from build123d import *

# Parameters (mm, degrees)
BOSS_EXTRUDE2_DEPTH      = 5
BOSS_EXTRUDE2_DEPTH_BACK = 5
CUT_EXTRUDE1_DEPTH       = 33.786759245
CUT_EXTRUDE1_DEPTH_BACK  = 33.786759245
SKETCH2_R                = 2
BOSS_EXTRUDE3_DEPTH      = 5
BOSS_EXTRUDE3_DEPTH_BACK = 5
SKETCH3_W                = 8
SKETCH3_H                = 1.5
CUT_EXTRUDE2_DEPTH       = 32.24718732
CUT_EXTRUDE2_DEPTH_BACK  = 32.24718732
SKETCH4_R                = 2
FILLET1_R                = 3


with BuildPart() as part:
    # Sketch1 → Boss-Extrude2 (new, two sides: drawn at the far end of the back side and taken through both)
    with BuildSketch(Plane.XY.offset(-BOSS_EXTRUDE2_DEPTH_BACK)):
        with BuildLine():
            Line((-16.929532322, 1.5), (-24.929532322, 1.5))
            Line((-24.929532322, 1.5), (-24.929532322, 3.5))
            Line((-24.929532322, 3.5), (-17.840130641, 3.5))
            ThreePointArc((-17.840130641, 3.5), (-10.970967291, 14.01498524), (1.215, 17.05678091))
            ThreePointArc((1.215, 17.05678091), (17.1, 0), (1.215, -17.05678091))
            ThreePointArc((1.215, -17.05678091), (-10.970967291, -14.01498524), (-17.840130641, -3.5))
            Line((-17.840130641, -3.5), (-24.929532322, -3.5))
            Line((-24.929532322, -3.5), (-24.929532322, -1.5))
            Line((-24.929532322, -1.5), (-16.929532322, -1.5))
            ThreePointArc((-16.929532322, -1.5), (-10.970813778, -12.51330782), (1.095, -15.862249998))
            ThreePointArc((1.095, -15.862249998), (15.9, 0), (1.095, 15.862249998))
            ThreePointArc((1.095, 15.862249998), (-10.970813778, 12.51330782), (-16.929532322, 1.5))
        make_face()
    extrude(amount=BOSS_EXTRUDE2_DEPTH + BOSS_EXTRUDE2_DEPTH_BACK)

    # Sketch2 → Cut-Extrude1 (cut, two sides: drawn at the far end of the back side and taken through both)
    with BuildSketch(Plane(origin=(0, 3.5, 0), x_dir=(1, 0, 0), z_dir=(0, 1, 0)).offset(-CUT_EXTRUDE1_DEPTH_BACK)):
        with Locations(Location((-21.429532322, 0, 0), (0, 0, 180))):
            Circle(SKETCH2_R)
    extrude(amount=CUT_EXTRUDE1_DEPTH + CUT_EXTRUDE1_DEPTH_BACK, mode=Mode.SUBTRACT)

    # Sketch3 → Boss-Extrude3 (add, two sides: drawn at the far end of the back side and taken through both)
    with BuildSketch(Plane.XY.offset(-BOSS_EXTRUDE3_DEPTH_BACK)):
        with Locations((21.083544714, 0)):
            Rectangle(SKETCH3_W, SKETCH3_H)
    extrude(amount=BOSS_EXTRUDE3_DEPTH + BOSS_EXTRUDE3_DEPTH_BACK)

    # Sketch4 → Cut-Extrude2 (cut, two sides: drawn at the far end of the back side and taken through both)
    with BuildSketch(Plane(origin=(0, 0.75, 0), x_dir=(1, 0, 0), z_dir=(0, 1, 0)).offset(-CUT_EXTRUDE2_DEPTH_BACK)):
        with Locations(Location((21.083544714, 0, 0), (0, 0, 180))):
            Circle(SKETCH4_R)
    extrude(amount=CUT_EXTRUDE2_DEPTH + CUT_EXTRUDE2_DEPTH_BACK, mode=Mode.SUBTRACT)

    # Fillet1
    fillet1_edges = [part.edges().sort_by_distance(p)[0] for p in [
        (-24.929532322, -2.5, -5),
        (-24.929532322, -2.5, 5),
        (-24.929532322, 2.5, 5),
        (-24.929532322, 2.5, -5),
        (25.083544714, 0, -5),
        (25.083544714, 0, 5),
    ]]
    fillet(fillet1_edges, radius=FILLET1_R)


solid = part.part
Could you check a few things on this model? Use its own coordinates, in mm. A direction names the side the tool comes from. Give positions to 0.01 mm unless a question says otherwise; leave off trailing zeros. Order: outer loops, then holes, each group sorted by start corner. A loop starts at its lowest first (then second) coordinate and runs counter-clockwise, first axis right, second up. Notation, with made-up numbers: (66, 38) -> (113, 38) arc R23 ccw to (113, 70) -> close; hole circle Ø8 at (-37.75, -28). An arc over 180 degrees is marked (long way). Answer in a Markdown table with one row per item. Add a question column.
Item 1: Imagine slicing it at B-B (z = 0). List the corners of the cut face in (x, y) for me (3 decimals).
Item 2: For faces 1 (the cylindrical face through (15.896, -0.334, -0.07)), 2 (the flat face through (-19, -1.5, 0)), 3 (the flat face through (-21.3, -3.5, 2.2)), 4 (the flat face through (-19, 3.5, 0)), which set-ups out of +Z, -Z, +X, -X, +Y, -Y let a thin tool reach every point of the face, with its end or its side?
Item 3: Imagine slicing it at D-D (y = 15). List the corners of the cut face in (x, z) for me, and give its area (3 significant figures).
Item 4: Please list where these lines run through material, in increasing order: probe 1 along X at (y, z) = (-2.2, 0); probe 2 along X at (y, z) = (-2.55, 0); probe 3 along Y at (x, z) = (1, 0.75).
Item 5: Imagine slicing it at C-C (x = 9.5). List the corners of the cut face in (y, z) for me.
Item 6: I'm going to push flat-ended pins straight in: P1, Ø10, axis at x = 4.5, y = 7, coming from the -Z side; P2, Ø4, axis at x = 19.5, z = -1.5, coming from the +Y side; P3, Ø5, axis at x = 21.08, z = 0, coming from the -Y side; P4, Ø3, axis at x = 13, z = 3, coming from the +Y side. Where does each tip first touch, or does it pass through?
Item 7: Imagine slicing it at A-A (y = 0). List the corners of the cut face in (x, z) for me.
Item 8: We'd pull the mould along Z, two halves only. Please class faces 5 (the cylindrical face through (23.08, -0.01, 0.09)), 6 (the flat face through (-24.93, -3, 0)), 7 (the cylindrical face through (-24.03, 2.51, -4.14)): pulls with the +Z half, pulls with the -Z half, needs draft (parallel to the pull), parting line crosses it, or undercut.
Result:
| question | item | result |
|---|---|---|
| 1 | outline | (-24.93, -3.5) -> (-23.43, -3.5) -> (-23.43, -1.5) -> (-24.93, -1.5) -> close; (-24.93, 1.5) -> (-23.43, 1.5) -> (-23.43, 3.5) -> (-24.93, 3.5) -> close; (-19.43, -3.5) -> (-17.84, -3.5) arc R17.2 ccw to (1.215, -17.057) arc R17.1 ccw to (17.084, -0.75) -> (19.084, -0.75) -> (19.084, 0.75) -> (17.084, 0.75) arc R17.1 ccw to (1.215, 17.057) arc R17.2 ccw to (-17.84, 3.5) -> (-19.43, 3.5) -> (-19.43, 1.5) -> (-16.93, 1.5) arc R16 cw to (1.095, 15.862) arc R15.9 cw to (1.095, -15.862) arc R16 cw to (-16.93, -1.5) -> (-19.43, -1.5) -> close; (23.084, -0.75) -> (25.084, -0.75) -> (25.084, 0.75) -> (23.084, 0.75) -> close |
| 2 | face 1 | +Z, -Z |
| 2 | face 2 | +Z, -Z, -X |
| 2 | face 3 | +Z, -Z, -X, -Y |
| 2 | face 4 | +Z, -Z, -X, +Y |
| 3 | outline | (-9.42, -5) -> (-6.57, -5) -> (-6.57, 5) -> (-9.42, 5) -> close; (5.27, -5) -> (8.21, -5) -> (8.21, 5) -> (5.27, 5) -> close |
| 3 | area | 57.9 mm2 |
| 4 | probe 1 | -24.93 to -23.43, -19.43 to -16.85, 15.75 to 16.96 |
| 4 | probe 2 | -24.93 to -23.43, -19.43 to -16.8, 15.69 to 16.91 |
| 4 | probe 3 | -17.08 to -15.87, 15.87 to 17.08 |
| 5 | outline | (-14.22, -5) -> (-12.75, -5) -> (-12.75, 5) -> (-14.22, 5) -> close; (12.75, -5) -> (14.22, -5) -> (14.22, 5) -> (12.75, 5) -> close |
| 6 | P1 | through |
| 6 | P2 | y = 0.75 |
| 6 | P3 | y = -0.75 |
| 6 | P4 | y = 12.66 |
| 7 | outline | (15.9, -5) -> (22.08, -5) arc R3 ccw to (25.08, -2) -> (25.08, 2) arc R3 ccw to (22.08, 5) -> (15.9, 5) -> close; hole circle Ø4 at (21.08, 0) |
| 8 | face 5 | undercut |
| 8 | face 6 | needs draft |
| 8 | face 7 | pulls with the -Z half |
